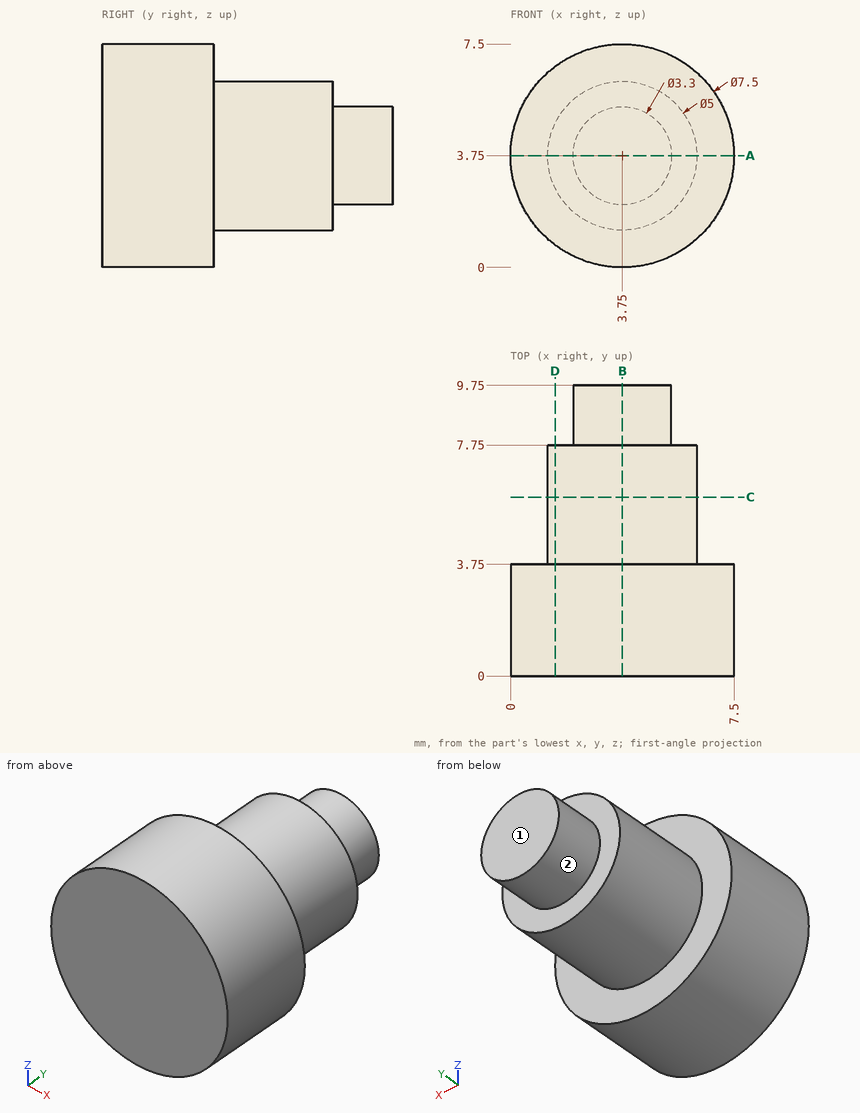
Print and shaded views of the part. All mm, measured from the part's lowest x, y and z. A direction names the side the tool comes from. Round coordinates to 2 decimals unless told otherwise and drop trailing zeros. Write each loop counter-clockwise with the first axis right and the second up, starting at its lowest first coordinate (ties: lowest second). Pieces come first, ordered by that corner, then holes. Notation, with made-up numbers: M -31.5,59 L -16.5,59 A13 ccw -16.5,69 Z; hole C 43,54.5 d4. An arc over 180 degrees is marked long. Use a Markdown table: item, result. Add a question column.
1. Slice it at C-C on y = 6. Give the cut face in (x, z), then the cut area to 3 significant figures.
2. Drill centre lines: probe 1 along Y at (x, z) = (1.25, 3); probe 2 along Y at (x, z) = (3.75, 1.5); probe 3 along X at (y, z) = (2.75, 5.5). Where is each one in solid material? Low to high.
3. Slice it at D-D on x = 1.5. Give the cut face in (y, z), then the cut area to 3 significant figures.
4. Slice it at A-A on z = 3.75. Give the cut face in (x, y), then the cut area to 3 significant figures.
5. 3-axis set-ups, long thin cutter, end or side, ignore diameter. For the marked faces 1 and 2: which of +Z, -Z, +X, -X, +Y, -Y reach the whole face in a straight line?
6. Flat gauge pins, fed straight in: P1, Ø3, axis at x = 4, z = 3.5, coming from the -Y side; P2, Ø1, axis at y = 2.5, z = 3, coming from the -X side; P3, Ø3, axis at x = 5.5, y = 7, coming from the -Z side. Where does each tip first touch, or does it go through?
7. Slice it at B-B on x = 3.75. Give the cut face in (y, z), then the cut area to 3 significant figures.
Reply:
| question | item | result |
|---|---|---|
| 1 | outline | C 3.75,3.75 d5 |
| 1 | area | 19.6 mm^2 |
| 2 | probe 1 | y = 0 to 3.75 |
| 2 | probe 2 | y = 0 to 7.75 |
| 2 | probe 3 | x = 0.43 to 7.07 |
| 3 | outline | M 0,0.75 L 3.75,0.75 L 3.75,2.66 L 7.75,2.66 L 7.75,4.84 L 3.75,4.84 L 3.75,6.75 L 0,6.75 Z |
| 3 | area | 31.2 mm^2 |
| 4 | outline | M 0,0 L 7.5,0 L 7.5,3.75 L 6.25,3.75 L 6.25,7.75 L 5.4,7.75 L 5.4,9.75 L 2.1,9.75 L 2.1,7.75 L 1.25,7.75 L 1.25,3.75 L 0,3.75 Z |
| 4 | area | 54.7 mm^2 |
| 5 | face 1 | +Z, -Z, +X, -X, +Y |
| 5 | face 2 | +Y |
| 6 | P1 | stops at y = 0 |
| 6 | P2 | stops at x = 0.01 |
| 6 | P3 | stops at z = 1.26 |
| 7 | outline | M 0,0 L 3.75,0 L 3.75,1.25 L 7.75,1.25 L 7.75,2.1 L 9.75,2.1 L 9.75,5.4 L 7.75,5.4 L 7.75,6.25 L 3.75,6.25 L 3.75,7.5 L 0,7.5 Z |
| 7 | area | 54.7 mm^2 |
